For this review, take the finished solid that the model builds, in its own axes (mm). Coordinates: 2 decimals unless noted, no trailing zeros. Loops run counter-clockwise (first coordinate to the right, second up) from the corner with the lowest first, then second, coordinate; pieces in that order, holes last. Notation, with made-up numbers: (26.5, 3) -> (47.5, 3) arc R20 ccw to (47.5, 31) -> close; hole circle Ø2 at (-28.75, -16). An arc over 180 degrees is marked (long way). Answer in a Markdown table with one row per item.
from build123d import *

# Parameters (mm, degrees)
F1_DEPTH = 25
F2_R     = 10


with BuildPart() as f1:
    # F0 (on Top) → F1 (new body)
    with BuildSketch(Plane.XY):
        with BuildLine():
            ThreePointArc((-16.4, 11.447270417), (-31.325290702, 0.2209930836), (-50, 0))
            ThreePointArc((-50, 0), (41, -28.6181760425), (-17.24, 46.9338087097))
            ThreePointArc((-17.24, 46.9338087097), (-11.0084011763, 29.3281056165), (-16.4, 11.447270417))
        make_face()
        with BuildLine():
            ThreePointArc((27.3, -8.5854528128), (7.8, -22.894540834), (0, 0))
            ThreePointArc((0, 0), (16.8, 5.7236352085), (27.3, -8.5854528128))
        make_face(mode=Mode.SUBTRACT)
    extrude(amount=F1_DEPTH)

    # F2
    f2_edges = [f1.edges().sort_by_distance(p)[0] for p in [
        (-50, 0, 12.5),
        (-17.24, 46.933809, 12.5),
    ]]
    fillet(f2_edges, radius=F2_R)


solid = f1.part
Item 1: Take a section at C-C, the plane x = 43.5. State the section outline as (y, z) points.
Worked answers:
| item | result |
|---|---|
| outline | (-24.65, 0) -> (24.65, 0) -> (24.65, 25) -> (-24.65, 25) -> close |
Item 2: Insertion check: pin 1 (2 mm diameter, centred on x = 19.5, z = 7.5, fed in from -Y); pin 2 (3 mm diameter, centred on y = 12, z = 16, fed in from -X); pin 3 (6 mm diameter, centred on x = 2, y = 33, fed in from -Z); pin 4 (10 mm diameter, centred on x = 16, z = 7, fed in from -Y) (3 decimals). Each pin has a flat end and moves straight along its axis. Give the tip position at first contact, or say it passes through.
Worked answers:
| item | result |
|---|---|
| pin 1 | y = -46.45 |
| pin 2 | x = -17.09 |
| pin 3 | z = 0 |
| pin 4 | y = -48.775 |
Item 3: Take a section at A-A, the plane y = 0. State the section outline as (x, z) points.
Worked answers:
| item | result |
|---|---|
| outline | (-32, 0) -> (0, 0) -> (0, 25) -> (-32, 25) -> close; (24.6, 0) -> (50, 0) -> (50, 25) -> (24.6, 25) -> close |
Item 4: Take a section at D-D, the plane y = -39. State the section outline as (x, z) points.
Worked answers:
| item | result |
|---|---|
| outline | (-31.29, 0) -> (31.29, 0) -> (31.29, 25) -> (-31.29, 25) -> close |
Item 5: Take a section at B-B, the plane x = 12.3. State the section outline as (y, z) points, and give its area (3 significant figures).
Worked answers:
| item | result |
|---|---|
| outline | (-48.46, 0) -> (-23.59, 0) -> (-23.59, 25) -> (-48.46, 25) -> close; (6.41, 0) -> (48.46, 0) -> (48.46, 25) -> (6.41, 25) -> close |
| area | 1,670 mm² |
Item 6: The part is to be moulded in two halves that separate along Y. For faces 1 (the cylindrical face through (24.966, -16.622, 12.325)), 2 (the cylindrical face through (40, -30, 12)), 3 (the flat face through (0, 1, 25)), say which applies: +Y half, -Y half, draft (parallel to the pull), parting line (faces both ways), or undercut.
Worked answers:
| item | result |
|---|---|
| face 1 | undercut |
| face 2 | parting line |
| face 3 | draft |
Item 7: For L1, parallel to Y at x = 12.3, z = 14; L2, parallel to Y at x = 8, z = 23 (3 decimals); L3, parallel to X at y = -39.5, z = 7, list the stretches that pass through material, from the lowest coordinate up.
Worked answers:
| item | result |
|---|---|
| L1 | -48.46 to -23.59, 6.41 to 48.46 |
| L2 | -49.356 to -22.956, 5.785 to 49.356 |
| L3 | -30.66 to 30.66 |
